```python
from build123d import *

# Parameters (mm, degrees)
F1_DEPTH = 12.7
F2_R     = 0.635


with BuildPart() as f1:
    # F0 (on Front) → F1 (new body)
    with BuildSketch(Plane.XZ):
        with BuildLine():
            Line((4.445, 3.81), (29.21, 3.81))
            Line((29.21, 3.81), (29.21, 6.35))
            Line((29.21, 6.35), (3.666174, 6.35))
            ThreePointArc((3.666174, 6.35), (-2.683826, 4.648523), (-7.332348, 0))
            Line((-7.332348, 0), (-20.104261, -22.121602))
            Line((-20.104261, -22.121602), (-17.904557, -23.391602))
            Line((-17.904557, -23.391602), (-5.522057, -1.944483))
            ThreePointArc((-5.522057, -1.944483), (-5.136481, -1.64862), (-4.654631, -1.712057))
            Line((-4.654631, -1.712057), (0.844631, -4.887057))
            ThreePointArc((0.844631, -4.887057), (1.140494, -5.272633), (1.077057, -5.754483))
            Line((1.077057, -5.754483), (-11.305443, -27.201602))
            Line((-11.305443, -27.201602), (-9.105739, -28.471602))
            Line((-9.105739, -28.471602), (3.666174, -6.35))
            Line((3.666174, -6.35), (29.21, -6.35))
            Line((29.21, -6.35), (29.21, -3.81))
            Line((29.21, -3.81), (4.445, -3.81))
            ThreePointArc((4.445, -3.81), (3.995987, -3.624013), (3.81, -3.175))
            Line((3.81, -3.175), (3.81, 3.175))
            ThreePointArc((3.81, 3.175), (3.995987, 3.624013), (4.445, 3.81))
        make_face()
    extrude(amount=F1_DEPTH)

    # F2
    f2_edges = [f1.edges().sort_by_distance(p)[0] for p in [
        (-2.719782, -12.7, -17.410801),
        (16.438087, -12.7, -6.35),
        (29.21, -12.7, -5.08),
        (16.8275, -12.7, -3.81),
        (3.995987, -12.7, -3.624013),
        (3.81, -12.7, 0),
        (3.995987, -12.7, 3.624013),
        (16.8275, -12.7, 3.81),
        (29.21, -12.7, 5.08),
        (16.438087, -12.7, 6.35),
        (-2.683826, -12.7, 4.648523),
        (-13.718305, -12.7, -11.060801),
        (-19.004409, -12.7, -22.756602),
        (-11.713307, -12.7, -12.668042),
        (-5.136481, -12.7, -1.64862),
        (-1.905, -12.7, -3.299557),
        (1.140494, -12.7, -5.272633),
        (-5.114193, -12.7, -16.478042),
        (-10.205591, -12.7, -27.836602),
        (29.21, -6.35, 3.81),
        (29.21, -6.35, 6.35),
        (29.21, 0, 5.08),
        (29.21, -6.35, -6.35),
        (29.21, -6.35, -3.81),
        (29.21, 0, -5.08),
        (-9.105739, -6.35, -28.471602),
        (3.666174, -6.35, -6.35),
        (-2.719782, 0, -17.410801),
        (16.438087, 0, -6.35),
        (16.8275, 0, -3.81),
        (3.995987, 0, -3.624013),
        (3.81, 0, 0),
        (3.995987, 0, 3.624013),
        (16.8275, 0, 3.81),
        (16.438087, 0, 6.35),
        (-2.683826, 0, 4.648523),
        (-13.718305, 0, -11.060801),
        (-19.004409, 0, -22.756602),
        (-11.713307, 0, -12.668042),
        (-5.136481, 0, -1.64862),
        (-1.905, 0, -3.299557),
        (1.140494, 0, -5.272633),
        (-5.114193, 0, -16.478042),
        (-10.205591, 0, -27.836602),
        (-11.305443, -6.35, -27.201602),
        (-20.104261, -6.35, -22.121602),
        (-17.904557, -6.35, -23.391602),
    ]]
    fillet(f2_edges, radius=F2_R)


solid = f1.part
```
Model file for the job. Use its own axes, mm. A direction names the side the tool comes from. Round coordinates to 2 decimals unless told otherwise and drop trailing zeros. Write each loop counter-clockwise with the first axis right and the second up, starting at its lowest first coordinate (ties: lowest second). Pieces come first, ordered by that corner, then holes. Notation, with made-up numbers: (69.5, 74) - (111.5, 74) arc R23 ccw to (111.5, 105) - close; hole circle Ø2 at (54.5, 82). An arc over 180 degrees is marked (long way). Use CSV: the item, a comma, the result in double quotes. Start each with the question number.
Item 1: Two-plate mould, pull along X, no slides. Class faces 1 (the face through (-11.63, -12.51, -12.16)), 2 (the face through (-2.603, -6.27, 4.695)), 3 (the face through (16, -6, -6.35)): released by +X, released by -X, zero draft, split by the parting line, or undercut.
Item 2: Pin check, flat tips, straight feed: P1, Ø4, axis at x = 8, y = -5.5, coming from the -Z side; P2, Ø4, axis at y = -8, z = -13.5, coming from the -X side; P3, Ø7, axis at y = -9, z = -0.5, coming from the +X side; P4, Ø8, axis at x = -11.5, z = -16, coming from the -Y side. Stop position of each tip, or through.
Item 3: Band-saw the part on A-A (x = 19). Write the cut outline in (y, z) (3 decimals), and give its area (3 significant figures).
Item 4: Drill centre lines: L1, parallel to Z at x = 5, y = -1; L2, parallel to X at y = -1, z = -7.5. Where is each one in solid material? Low to high. Write a range as [from, to].
Item 5: Tool access for faces 4 (the face through (-11.63, -0.19, -12.16)), 5 (the face through (-1.78, -12.51, -3.16)), 6 (the face through (-1.94, -6.27, -3.28)): list every direction of +Z, -Z, +X, -X, +Y, -Y with a clear straight run to the whole face (end or side of a thin tool).
Checked values:
1,face 1,"undercut"
1,face 2,"released by -X"
1,face 3,"zero draft"
2,P1,"stops at z = -6.35"
2,P2,"stops at x = -16.28"
2,P3,"stops at x = 29.03"
2,P4,"stops at y = -12.7"
3,outline,"(-12.7, -5.715) arc R0.635 ccw to (-12.065, -6.35) - (-0.635, -6.35) arc R0.635 ccw to (0, -5.715) - (0, -4.445) arc R0.635 ccw to (-0.635, -3.81) - (-12.065, -3.81) arc R0.635 ccw to (-12.7, -4.445) - close; (-12.7, 4.445) arc R0.635 ccw to (-12.065, 3.81) - (-0.635, 3.81) arc R0.635 ccw to (0, 4.445) - (0, 5.715) arc R0.635 ccw to (-0.635, 6.35) - (-12.065, 6.35) arc R0.635 ccw to (-12.7, 5.715) - close"
3,area,"63.8 mm²"
4,L1,"z = [-6.35, -3.81], [3.81, 6.35]"
4,L2,"x = [-11.66, -8.73], [0.07, 3]"
5,face 4,"+Y"
5,face 5,"-Y"
5,face 6,"+Y, -Y"
